from build123d import *

# Parameters (mm, degrees)
SKETCH1_W           = 161
SKETCH1_H           = 82.5
BOSS_EXTRUDE1_DEPTH = 35
FILLET1_R           = 10
BOSS_EXTRUDE2_DEPTH = 1
BOSS_EXTRUDE3_START = 1
BOSS_EXTRUDE3_DEPTH = 1
SKETCH4_W           = 146.0174604
SKETCH4_H           = 12.670298151
CUT_EXTRUDE1_DEPTH  = 1
SKETCH6_W           = 20.834184422
SKETCH6_H           = 10.266465629
BOSS_EXTRUDE5_DEPTH = 0.5
SKETCH7_R           = 8.605932771
BOSS_EXTRUDE6_DEPTH = 0.5


with BuildPart() as part:
    # Sketch1 → Boss-Extrude1 (new body)
    with BuildSketch(Plane(origin=(0, 0, 0), x_dir=(1, 0, 0), z_dir=(0, 1, 0))):
        Rectangle(SKETCH1_W, SKETCH1_H)
    extrude(amount=BOSS_EXTRUDE1_DEPTH)

    # Fillet1
    fillet1_edges = [part.edges().sort_by_distance(p)[0] for p in [
        (0, 35, -41.25),
        (0, 0, -41.25),
        (0, 0, 41.25),
        (0, 35, 41.25),
    ]]
    fillet(fillet1_edges, radius=FILLET1_R)

    # Sketch2 → Boss-Extrude2 (add)
    with BuildSketch(Plane(origin=(80.5, 0, 0), x_dir=(0, 0, -1), z_dir=(1, 0, 0))):
        with BuildLine():
            Line((38.25, 10), (38.25, 25))
            ThreePointArc((38.25, 25), (36.199747468, 29.949747468), (31.25, 32))
            Line((31.25, 32), (-31.25, 32))
            ThreePointArc((-31.25, 32), (-36.199747468, 29.949747468), (-38.25, 25))
            Line((-38.25, 25), (-38.25, 10))
            ThreePointArc((-38.25, 10), (-36.199747468, 5.050252532), (-31.25, 3))
            Line((-31.25, 3), (31.25, 3))
            ThreePointArc((31.25, 3), (36.199747468, 5.050252532), (38.25, 10))
        make_face()
    extrude(amount=BOSS_EXTRUDE2_DEPTH)

    # Sketch3 → Boss-Extrude3 (add)
    with BuildSketch(Plane.ZY.offset(80.5).offset(BOSS_EXTRUDE3_START)):
        with BuildLine():
            Line((31.25, 32), (-31.25, 32))
            ThreePointArc((-31.25, 32), (-36.199747468, 29.949747468), (-38.25, 25))
            Line((-38.25, 25), (-38.25, 10))
            ThreePointArc((-38.25, 10), (-36.199747468, 5.050252532), (-31.25, 3))
            Line((-31.25, 3), (31.25, 3))
            ThreePointArc((31.25, 3), (36.199747468, 5.050252532), (38.25, 10))
            Line((38.25, 10), (38.25, 25))
            ThreePointArc((38.25, 25), (36.199747468, 29.949747468), (31.25, 32))
        make_face()
    extrude(amount=-BOSS_EXTRUDE3_DEPTH)

    # Sketch4 → Cut-Extrude1 (cut)
    with BuildSketch(Plane(origin=(0, 35, 0), x_dir=(1, 0, 0), z_dir=(0, 1, 0))):
        with Locations((0.540805409, -23.022858836)):
            Rectangle(SKETCH4_W, SKETCH4_H)
    extrude(amount=-CUT_EXTRUDE1_DEPTH, mode=Mode.SUBTRACT)

    # Sketch6 → Boss-Extrude5 (add)
    with BuildSketch(Plane(origin=(0, 34, 0), x_dir=(1, 0, 0), z_dir=(0, 1, 0))):
        with Locations((0, -22.722377564)):
            Rectangle(SKETCH6_W, SKETCH6_H)
    extrude(amount=BOSS_EXTRUDE5_DEPTH)

    # Sketch7 → Boss-Extrude6 (add)
    with BuildSketch(Plane.ZY.offset(81.5)):
        with Locations((0, 17.304485336)):
            Circle(SKETCH7_R)
    extrude(amount=BOSS_EXTRUDE6_DEPTH)


solid = part.part
Geometry check sheet. Reference: the model listing, model coordinates, mm. A direction names the side the tool comes from. Give positions to 0.01 mm unless a question says otherwise; leave off trailing zeros. Loops run counter-clockwise (first coordinate to the right, second up) from the corner with the lowest first, then second, coordinate; pieces in that order, holes last.
(1) Section check A-A on x = 23.5. Record the cut outline in (y, z).
From the geometry:
outline: (0, -31.25) arc R10 ccw to (10, -41.25) - (25, -41.25) arc R10 ccw to (35, -31.25) - (35, 16.69) - (34, 16.69) - (34, 29.36) - (35, 29.36) - (35, 31.25) arc R10 ccw to (25, 41.25) - (10, 41.25) arc R10 ccw to (0, 31.25) - close
(2) Thickness scan on L1, parallel to X at y = 28.5, z = 34; L2, parallel to Y at x = 7.5, z = 26.5; L3, parallel to X at y = 33, z = 4.5. Record the ranges inside material, lowest first.
From the geometry:
L1: x = -81.5 to 81.5
L2: y = 0 to 34.5
L3: x = -80.5 to 80.5
(3) Depth check by flat-ended pin: pin 1 Ø8 at (x, z) = (2, 24) entering from +Y; pin 2 Ø0.8 at (x, y) = (81, 19.5) entering from +Z; pin 3 Ø1.5 at (y, z) = (19, 30) entering from -X. Enter the tip coordinate at first touch or a pass-through.
From the geometry:
pin 1: stops at y = 34.5
pin 2: stops at z = 38.25
pin 3: stops at x = -81.5
(4) Set-up check for faces 1 (the cylindrical face through (80.99, 5.1, 36.25)), 2 (the cylindrical face through (-81.01, 5, 36.15)), 3 (the flat face through (80.5, 33, 0)), 4 (the flat face through (-80.5, 33, 0)): record each of +Z, -Z, +X, -X, +Y, -Y from which the full face is reachable in a straight line by a thin tool's end or side.
From the geometry:
face 1: +Z, +X, -Y
face 2: +Z, -X, -Y
face 3: +X
face 4: -X
(5) Release check for a two-part mould opening along X. For faces 5 (the flat face through (0, 34.5, 23)), 6 (the cylindrical face through (1.13, 31.99, 38.4)), 7 (the flat face through (-82, 17, 0)) record: released by +X, released by -X, zero draft, split by the parting line, or undercut.
From the geometry:
face 5: undercut
face 6: zero draft
face 7: released by -X
